CAD build for the part. Positions are in the model's coordinates, mm. Face numbers are marked on the shaded views. Give positions to 0.01 mm unless a question says otherwise; leave off trailing zeros. Write each loop counter-clockwise with the first axis right and the second up, starting at its lowest first coordinate (ties: lowest second). Pieces come first, ordered by that corner, then holes. Notation, with made-up numbers: (79.5, -40) -> (89.5, -40) arc R23 cw to (89.5, -19) -> close; hole circle Ø2 at (4, 29.5). An arc over 180 degrees is marked (long way). Answer as a JSON object with one key per item and string values.
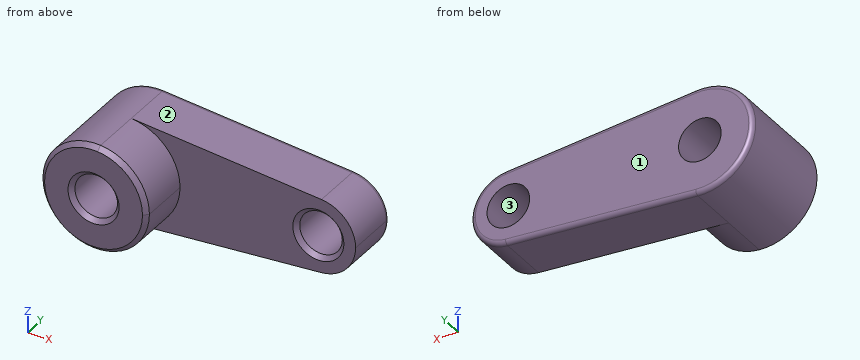
```python
from build123d import *

# Parameters (mm, degrees)
F0_R     = 25.4
F1_DEPTH = 63.5
F2_DEPTH = 127
F3_SIZE  = 5.08
F4_R     = 5.08


with BuildPart() as f1:
    # F0 (on Front) → F1 (new body)
    with BuildSketch(Plane.XZ):
        with BuildLine():
            ThreePointArc((5.291667, -63.27913), (46.734735, -42.989703), (63.5, 0))
            ThreePointArc((63.5, 0), (46.734735, 42.989703), (5.291667, 63.27913))
            ThreePointArc((5.291667, 63.27913), (-63.5, 0), (5.291667, -63.27913))
        make_face()
        Circle(F0_R, mode=Mode.SUBTRACT)
        with BuildLine():
            ThreePointArc((5.291667, 63.27913), (46.734735, 42.989703), (63.5, 0))
            ThreePointArc((63.5, 0), (46.734735, -42.989703), (5.291667, -63.27913))
            Line((5.291667, -63.27913), (232.304167, -44.295391))
            ThreePointArc((232.304167, -44.295391), (184.15, 0), (232.304167, 44.295391))
            Line((232.304167, 44.295391), (5.291667, 63.27913))
        make_face()
        with BuildLine():
            ThreePointArc((273.05, 0), (261.314314, 30.092792), (232.304167, 44.295391))
            ThreePointArc((232.304167, 44.295391), (184.15, 0), (232.304167, -44.295391))
            ThreePointArc((232.304167, -44.295391), (261.314314, -30.092792), (273.05, 0))
        make_face()
        with Locations((228.6, 0)):
            Circle(F0_R, mode=Mode.SUBTRACT)
    extrude(amount=F1_DEPTH)

    # F0 (on Front) → F2 (join)
    with BuildSketch(Plane.XZ):
        with BuildLine():
            ThreePointArc((5.291667, -63.27913), (46.734735, -42.989703), (63.5, 0))
            ThreePointArc((63.5, 0), (46.734735, 42.989703), (5.291667, 63.27913))
            ThreePointArc((5.291667, 63.27913), (-63.5, 0), (5.291667, -63.27913))
        make_face()
        Circle(F0_R, mode=Mode.SUBTRACT)
    extrude(amount=F2_DEPTH)

    # F3
    f3_edges = [f1.edges().sort_by_distance(p)[0] for p in [
        (-25.4, -127, 0),
        (-5.291667, -127, 63.27913),
        (203.2, -63.5, 0),
    ]]
    chamfer(f3_edges, length=F3_SIZE)

    # F4
    f4_edges = [f1.edges().sort_by_distance(p)[0] for p in [
        (118.797917, 0, 53.78726),
        (118.797917, 0, -53.78726),
        (-63.5, 0, 0),
        (273.05, 0, 0),
    ]]
    fillet(f4_edges, radius=F4_R)


solid = f1.part
```
1) Slice it at C-C (z = -9). State how many separate pieces and enclosed holes the cut face has, then the cut area to 3 significant figures.
Model answer:
{"separate pieces": "3", "enclosed holes": "0", "area": "20,100 mm2"}
2) Mould opens along X. For the marked faces 1, 2 and 3 say: released by +X, released by -X, zero draft, split by the parting line, or undercut.
Model answer:
{"face 1": "zero draft", "face 2": "released by +X", "face 3": "undercut"}
3) Slice it at B-B (y = -97). List the corners of the cut face in (x, z).
Model answer:
{"outline": "circle Ø127 at (0, 0); hole circle Ø50.8 at (0, 0)"}
4) Slice it at A-A (y = -46.5). List the corners of the cut face in (x, z).
Model answer:
{"outline": "(5.29, -63.28) -> (232.3, -44.3) arc R44.45 ccw to (273.05, 0) arc R44.45 ccw to (232.3, 44.3) -> (5.29, 63.28) arc R63.5 ccw (long way) to start; hole circle Ø50.8 at (0, 0); hole circle Ø50.8 at (228.6, 0)"}
5) Pin check, flat tips, straight feed: pin 1 (4 mm diameter, centred on x = 113, y = -63.5, fed in from -Z); pin 2 (3 mm diameter, centred on x = 67, z = -39.5, fed in from -Y); pin 3 (10 mm diameter, centred on y = -86.5, z = -47.5, fed in from +X). Stop position of each tip, or through.
Model answer:
{"pin 1": "stops at z = -54.44", "pin 2": "stops at y = -63.5", "pin 3": "stops at x = 47.18"}
6) Wall check: probe 1 along Z at (x, y) = (0, -60); probe 2 along Y at (x, z) = (69, -34); probe 3 along X at (y, z) = (-119.5, 21). Give the ranges that are in metal, low to high.
Model answer:
{"probe 1": "z = -63.5 to -25.4, 25.4 to 63.5", "probe 2": "y = -63.5 to 0", "probe 3": "x = -59.93 to -14.29, 14.29 to 59.93"}
